Can you work these out from the model? Positions are in its coordinate system, mm. A direction names the side the tool comes from. Coordinates: 2 decimals unless noted, no trailing zeros. Order: outer loops, then holes, each group sorted by start corner. A loop starts at its lowest first (then second) coordinate and runs counter-clockwise, first axis right, second up. Notation, with made-up numbers: (29.25, -29) -> (61.25, -29) arc R20 ccw to (61.25, 4) -> close; hole circle Ø11 at (76, -7). An arc over 180 degrees is marked (long way). Write item = value, one per line.
```python
from build123d import *

# Parameters (mm, degrees)
SKETCH1_W               = 20.5
SKETCH1_H               = 8
BOSS_EXTRUDE1_DEPTH     = 3
CUT_EXTRUDE1_DEPTH      = 23.209232315
CUT_EXTRUDE1_DEPTH_BACK = 23.209232315
CUT_EXTRUDE2_DEPTH      = 23.209232315
CUT_EXTRUDE2_DEPTH_BACK = 23.209232315
SKETCH4_R               = 1.8
CUT_EXTRUDE3_DEPTH      = 0.8
SKETCH5_W               = 8
SKETCH5_H               = 1
BOSS_EXTRUDE2_DEPTH     = 2
FILLET1_R               = 4


with BuildPart() as part:
    # Sketch1 → Boss-Extrude1 (new body)
    with BuildSketch(Plane(origin=(0, 0, 0), x_dir=(1, 0, 0), z_dir=(0, 1, 0))):
        with Locations((10.25, 4)):
            Rectangle(SKETCH1_W, SKETCH1_H)
    extrude(amount=BOSS_EXTRUDE1_DEPTH)

    # Sketch2 → Cut-Extrude1 (cut, two sides: drawn at the far end of the back side and taken through both)
    with BuildSketch(Plane.XY.offset(-CUT_EXTRUDE1_DEPTH_BACK)):
        Polygon((0, 0), (0.6, 3), (0, 3), align=None)
        Polygon((20.5, 0), (19.9, 3), (20.5, 3), align=None)
    extrude(amount=CUT_EXTRUDE1_DEPTH + CUT_EXTRUDE1_DEPTH_BACK, mode=Mode.SUBTRACT)

    # Sketch3 → Cut-Extrude2 (cut, two sides: drawn at the far end of the back side and taken through both)
    with BuildSketch(Plane(origin=(0, 0, 0), x_dir=(0, 0, -1), z_dir=(1, 0, 0)).offset(-CUT_EXTRUDE2_DEPTH_BACK)):
        Polygon((0, 0), (0.6, 3), (0, 3), align=None)
        Polygon((8, 3), (7.4, 3), (8, 0), align=None)
    extrude(amount=CUT_EXTRUDE2_DEPTH + CUT_EXTRUDE2_DEPTH_BACK, mode=Mode.SUBTRACT)

    # Sketch4 → Cut-Extrude3 (cut)
    with BuildSketch(Plane.XZ):
        with Locations(Location((10.25000125, -3.75, 0), (0, 0, 270))):
            Circle(SKETCH4_R)
    extrude(amount=-CUT_EXTRUDE3_DEPTH, mode=Mode.SUBTRACT)

    # Sketch5 → Boss-Extrude2 (add)
    with BuildSketch(Plane.XZ):
        with Locations((10.250011, -7.5)):
            Rectangle(SKETCH5_W, SKETCH5_H)
    extrude(amount=BOSS_EXTRUDE2_DEPTH)

    # Fillet1
    # the kernel refuses this fillet: 4 mm, written as the material it takes off along each edge
    with BuildSketch(Plane(origin=(14.250011, -2, -16.660254038), x_dir=(0, 1, 0), z_dir=(0, 0, 1)), Plane(origin=(6.250011, -2, 1.660254038), x_dir=(0, 1, 0), z_dir=(0, 0, -1))) as fillet1_piece_1:
        with BuildLine():
            CenterArc((4, 3.464101615), FILLET1_R, 180, 60)
            Line((0, 3.464101615), (-0.08, 3.464101615))
            Line((-0.08, 3.464101615), (-0.08, 0))
            Line((-0.08, 0), (0, -0.08))
            ThreePointArc((0, -0.08), (1, -0.08), (1.96, -0.069282032))
            Line((1.96, -0.069282032), (2, 0))
        make_face()
    extrude(amount=18.320508076, mode=Mode.SUBTRACT)


solid = part.part
```
Item 1: I want a section at D-D, the plane z = -2.25. Please give me the cut outline in (x, y).
A:
outline = (0, 0) -> (9.26, 0) -> (9.26, 0.8) -> (11.24, 0.8) -> (11.24, 0) -> (20.5, 0) -> (19.9, 3) -> (0.6, 3) -> close
Item 2: For faces 1 (the flat face through (10, -1, -7)), 2 (the flat face through (10, -1, -8)), which set-ups out of +Z, -Z, +X, -X, +Y, -Y let a thin tool reach every point of the face, with its end or its side?
A:
face_1 = +Z, +X, -X, -Y
face_2 = -Z, +X, -X, +Y, -Y
Item 3: I want a section at C-C, the plane y = 1.9. Please give me the cut outline in (x, z).
A:
outline = (0.38, -7.62) -> (20.12, -7.62) -> (20.12, -0.38) -> (0.38, -0.38) -> close
Item 4: I'm going to push flat-ended pins straight in: P1, Ø4, axis at x = 7, z = -3, coming from the -Y side; P2, Ø1.1, axis at x = 10, z = -4.5, coming from the -Y side; P3, Ø3, axis at y = -1, z = -7, coming from the +X side; P4, Ø1, axis at x = 9, y = -1, coming from the +Z side. Where does each tip first touch, or does it pass through?
A:
P1 = 0
P2 = 0.8
P3 = 20.5
P4 = -7
Item 5: If I drill on probe 1 along Y at (x, z) = (9.5, -4); probe 2 along X at (y, z) = (0.6, -3.75); probe 3 along Y at (x, z) = (7, -1.75), over which ranges is the centre line in solid material (lowest first)?
A:
probe_1 = 0.8 to 3
probe_2 = 0.12 to 8.45, 12.05 to 20.38
probe_3 = 0 to 3
Item 6: I want a section at B-B, the plane z = -3.75. Please give me the cut outline in (x, y).
A:
outline = (0, 0) -> (8.45, 0) -> (8.45, 0.8) -> (12.05, 0.8) -> (12.05, 0) -> (20.5, 0) -> (19.9, 3) -> (0.6, 3) -> close
Item 7: I want a section at A-A, the plane y = 0.3. Please give me the cut outline in (x, z).
A:
outline = (0.06, -7.94) -> (20.44, -7.94) -> (20.44, -0.06) -> (0.06, -0.06) -> close; hole circle Ø3.6 at (10.25, -3.75)
Item 8: If we mould it in two halves opening along Z, with no side actions, what happens to faces 3 (the cylindrical face through (7.74, -1.48, -7.49)), 4 (the flat face through (10.1, 1.5, -7.7)), 5 (the cylindrical face through (9.561, 0.394, -5.413)), 6 (the flat face through (10, 0.8, -4))? For each: pulls with the +Z half, pulls with the -Z half, needs draft (parallel to the pull), parting line crosses it, or undercut.
A:
face_3 = needs draft
face_4 = pulls with the -Z half
face_5 = undercut
face_6 = undercut
